Design review of the part built by this model. Coordinates are the model's own, in mm. A direction names the side the tool comes from. Coordinates: 2 decimals unless noted, no trailing zeros. Write each loop counter-clockwise with the first axis right and the second up, starting at its lowest first coordinate (ties: lowest second). Pieces come first, ordered by that corner, then holes. Notation, with made-up numbers: (82.5, -15) - (94.5, -15) arc R22 cw to (94.5, 23) - close; hole circle Ø7 at (52, 35.5). An arc over 180 degrees is marked (long way). Answer as a JSON object with one key per item and string values.
```python
from build123d import *

# Parameters (mm, degrees)
CROQUIS1_R               = 35
SALIENTE_EXTRUIR15_DEPTH = 40


with BuildPart() as part:
    # Croquis1 → Saliente-Extruir15 (new body)
    with BuildSketch(Plane.XY):
        with BuildLine():
            Line((-14.686304328, 314.09938136), (73.062849976, 489.074174319))
            Line((73.062849976, 489.074174319), (55.185016864, 498.039835657))
            Line((55.185016864, 498.039835657), (-32.617627004, 318.343715137))
            ThreePointArc((-32.617627004, 318.343715137), (-56.321599928, 310.563610662), (-70.80460356, 290.249798518))
            add(Edge.make_bspline(
                [(-70.80460356, 290.249798518), (-421.705541448, 191.98441708), (-244.154369287, -146.862508424)],
                knots=[3.397241876, 3.397241876, 3.397241876, 5.223953064, 5.223953064, 5.223953064], degree=2, weights=[1, 0.611093045, 1]))
            Line((-244.154369287, -146.862508424), (-221.365281412, -146.862508424))
            add(Edge.make_bspline(
                [(-71.555520961, 269.187274007), (-401.226138708, 167.553458018), (-221.365281412, -146.862508424)],
                knots=[0.278811815, 0.278811815, 0.278811815, 2.122934595, 2.122934595, 2.122934595], degree=2, weights=[1, 0.604178825, 1]))
            ThreePointArc((-71.555520961, 269.187274007), (-7.826633559, 246.952527775), (-14.686304328, 314.09938136))
        make_face()
        with Locations((-32.617627004, 278.343715137)):
            Circle(CROQUIS1_R, mode=Mode.SUBTRACT)
    extrude(amount=SALIENTE_EXTRUIR15_DEPTH)


solid = part.part
```
(1) Take a section at A-A, the plane x = -41.5. Write out the cut boundary in (y, z), and give its area (3 significant figures).
Solved:
{"outline": "(239.34, 0) - (244.49, 0) - (244.49, 40) - (239.34, 40) - close; (312.2, 0) - (317.35, 0) - (317.35, 40) - (312.2, 40) - close", "area": "412 mm^2"}
(2) For pin 1 (3 mm diameter, centred on y = 376, z = 13.5, fed in from -X); pin 2 (5 mm diameter, centred on x = -209.5, z = 28, fed in from -Y); pin 3 (10 mm diameter, centred on x = -91.5, z = 14.5, fed in from -Y), all flat-tipped, find the tip position at first contact; note any pin that passes through.
Solved:
{"pin 1": "stops at x = -5.18", "pin 2": "stops at y = 162.1", "pin 3": "stops at y = 260"}
(3) Tool access review of faces 1 (the face through (64.249, 493.494, 19.72)), 2 (the face through (28.574, 400.362, 19.72)): name each direction out of +Z, -Z, +X, -X, +Y, -Y from which nothing blocks a thin tool from reaching the whole face with its end or side.
Solved:
{"face 1": "+Z, -Z, +X, +Y", "face 2": "+Z, -Z, +X"}
(4) To check wall thickness, follow line 1 (Y direction, x = -4, z = 30.5); line 2 (Y direction, x = -226.5, z = 28); line 3 (Y direction, x = -23.5, z = 34). State the ranges of each line that lie inside material, in increasing order. Write a range as from..to.
Solved:
{"line 1": "y = 250.4..258.19, 298.49..306.29, 335.41..376.91", "line 2": "y = -146.86..-137.48, 137.48..176.37", "line 3": "y = 239.4..244.55, 312.14..337"}
(5) Take a section at B-B, the plane x = 31. Write out the cut boundary in (y, z).
Solved:
{"outline": "(405.2, 0) - (448.54, 0) - (448.54, 40) - (405.2, 40) - close"}
(6) The part is to be moulded in two halves that separate along X. For faces 3 (the face through (11.9, 409.45, 19.72)), 4 (the face through (-8.719, 246.268, 19.72)), 5 (the face through (-194, 201, 0)), say which applies: pulls with the +X half, pulls with the -X half, needs draft (parallel to the pull), parting line crosses it, or undercut.
Solved:
{"face 3": "pulls with the -X half", "face 4": "undercut", "face 5": "needs draft"}
